```python
from build123d import *

# Parameters (mm, degrees)
SKETCH1_W                = 71
SKETCH1_H                = 80
BOSS_EXTRUDE1_DEPTH      = 10
SKETCH3_W                = 10
SKETCH3_H                = 10
CUT_EXTRUDE1_DEPTH       = 10
SKETCH5_W                = 28.158683969
SKETCH5_H                = 10
CUT_EXTRUDE3_DEPTH       = 10
CIRPATTERN1_COUNT        = 3
M6_CLEARANCE_HOLE1_D     = 6.3
CUT_EXTRUDE6_DEPTH       = 3
SKETCH11_R               = 1.55
CUT_EXTRUDE7_DEPTH       = 108.429046352
CIRPATTERN2_COUNT        = 3
CUT_EXTRUDE8_DEPTH       = 10
CUT_EXTRUDE9_DEPTH       = 10
CUT_EXTRUDE10_DEPTH      = 10
SKETCH15_W               = 111
SKETCH15_H               = 42
BOSS_EXTRUDE2_DEPTH      = 10
SKETCH22_W               = 15
SKETCH22_H               = 54
BOSS_EXTRUDE3_DEPTH      = 10
M4_CLEARANCE_HOLE1_D     = 4.5
M4_CLEARANCE_HOLE1_DEPTH = 30
M4_CLEARANCE_HOLE1_TIP   = 1.351936393
SKETCH26_W               = 47.7
SKETCH26_H               = 6
CUT_EXTRUDE13_DEPTH      = 10
CHAMFER1_SIZE            = 4
CHAMFER1_SIZE_2          = 6.92820323
SKETCH27_W               = 6.3
SKETCH27_H               = 6
CUT_EXTRUDE14_DEPTH      = 10
CHAMFER2_SIZE            = 6.92820323
CHAMFER2_SIZE_2          = 4
CUT_EXTRUDE15_DEPTH      = 10
CUT_EXTRUDE16_DEPTH      = 2.2
CUT_EXTRUDE17_DEPTH      = 10
M4_CLEARANCE_HOLE2_D     = 4.5
SKETCH33_W               = 30
SKETCH33_H               = 90
CUT_EXTRUDE18_DEPTH      = 138.189649755
SKETCH34_W               = 10
SKETCH34_H               = 22
BOSS_EXTRUDE4_DEPTH      = 5
SKETCH38_R               = 2.25
CUT_EXTRUDE20_DEPTH      = 41
CHAMFER3_SIZE            = 2


with BuildPart() as part:
    # Sketch1 → Boss-Extrude1 (new body)
    with BuildSketch(Plane.XY):
        with Locations((35.5, 40)):
            Rectangle(SKETCH1_W, SKETCH1_H)
    extrude(amount=BOSS_EXTRUDE1_DEPTH)

    # Sketch3 → Cut-Extrude1 (cut)
    with BuildSketch(Plane.XY.offset(10)):
        Polygon((25.580127019, 57.655444566), (16.919872981, 52.655444566), (11.919872981, 61.315698604), (20.580127019, 66.315698604), align=None)
        Polygon((11.919872981, 18.684301396), (20.580127019, 13.684301396), (25.580127019, 22.344555434), (16.919872981, 27.344555434), align=None)
        with Locations((52.5, 40)):
            Rectangle(SKETCH3_W, SKETCH3_H)
    extrude(amount=-CUT_EXTRUDE1_DEPTH, mode=Mode.SUBTRACT)

    # Sketch5 → Cut-Extrude3 (cut)
    with BuildSketch(Plane.XY.offset(10)):
        with Locations((71.579341985, 40)):
            Rectangle(SKETCH5_W, SKETCH5_H)
    cut_extrude3 = extrude(amount=-CUT_EXTRUDE3_DEPTH, mode=Mode.SUBTRACT)

    # CirPattern1: Cut-Extrude3 ×3 about axis
    cirpattern1_axis = Axis((30, 40, 10), (0, 0, -1))
    for i in range(1, CIRPATTERN1_COUNT):
        add(cut_extrude3.rotate(cirpattern1_axis, i * 360 / CIRPATTERN1_COUNT), mode=Mode.SUBTRACT)

    # M6 Clearance Hole1 (through all)
    with Locations(Plane.XY.offset(10)):
        with Locations((30, 40)):
            Hole(M6_CLEARANCE_HOLE1_D / 2)

    # Sketch10 → Cut-Extrude6 (cut)
    with BuildSketch(Plane.XY.offset(10)):
        Polygon((30, 45.773502692), (25, 42.886751346), (25, 37.113248654), (30, 34.226497308), (35, 37.113248654), (35, 42.886751346), align=None)
    extrude(amount=-CUT_EXTRUDE6_DEPTH, mode=Mode.SUBTRACT)

    # Sketch11 → Cut-Extrude7 (cut, through all)
    with BuildSketch(Plane.XZ):
        with Locations(Location((62.5, 5, 0), (0, 0, 270))):
            Circle(SKETCH11_R)
    cut_extrude7 = extrude(amount=-CUT_EXTRUDE7_DEPTH, mode=Mode.SUBTRACT)

    # CirPattern2: Cut-Extrude7 ×3 about axis
    cirpattern2_axis = Axis((30, 40, 7), (0, 0, 1))
    for i in range(1, CIRPATTERN2_COUNT):
        add(cut_extrude7.rotate(cirpattern2_axis, i * 360 / CIRPATTERN2_COUNT), mode=Mode.SUBTRACT)

    # Sketch12 → Cut-Extrude8 (cut)
    with BuildSketch(Plane.XY.offset(10)):
        Polygon((71, 0), (71, 25), (38.660254038, 25), (24.226497308, 0), align=None)
    cut_extrude8 = extrude(amount=-CUT_EXTRUDE8_DEPTH, mode=Mode.SUBTRACT)

    # Mirror1: Cut-Extrude8 across plane
    add(cut_extrude8.mirror(Plane(origin=(0, 40, 0), x_dir=(0, 0, 1), z_dir=(0, -1, 0))), mode=Mode.SUBTRACT)

    # Sketch13 → Cut-Extrude9 (cut)
    with BuildSketch(Plane.XY.offset(10)):
        Polygon((0, 61.961524227), (8.624364028, 47.023687548), (8.624364028, 32.976312452), (0, 18.038475773), align=None)
    extrude(amount=-CUT_EXTRUDE9_DEPTH, mode=Mode.SUBTRACT)

    # Sketch14 → Cut-Extrude10 (cut)
    with BuildSketch(Plane.XY.offset(10)):
        Polygon((-3.240381057, 12.425971147), (22.740381057, -2.574028853), (18.169872981, -10.490381057), (-7.810889132, 4.509618943), align=None)
    cut_extrude10 = extrude(amount=-CUT_EXTRUDE10_DEPTH, mode=Mode.SUBTRACT)

    # Mirror2: Cut-Extrude10 across plane
    add(cut_extrude10.mirror(Plane(origin=(0, 40, 0), x_dir=(0, 0, 1), z_dir=(0, -1, 0))), mode=Mode.SUBTRACT)

    # Sketch15 → Boss-Extrude2 (add)
    with BuildSketch(Plane.XY.offset(10)):
        with Locations((126.5, 40)):
            Rectangle(SKETCH15_W, SKETCH15_H)
    extrude(amount=-BOSS_EXTRUDE2_DEPTH)

    # Sketch22 → Boss-Extrude3 (add)
    with BuildSketch(Plane.XY.offset(10)):
        with Locations((174.5, 40)):
            Rectangle(SKETCH22_W, SKETCH22_H)
    extrude(amount=-BOSS_EXTRUDE3_DEPTH)

    # M4 Clearance Hole1
    with Locations(Plane(origin=(182, 0, 0), x_dir=(0, 0, -1), z_dir=(1, 0, 0))):
        with Locations((-5, 62.5), (-5, 17.5)):
            Hole(M4_CLEARANCE_HOLE1_D / 2, depth=M4_CLEARANCE_HOLE1_DEPTH)
            with Locations((0, 0, -(M4_CLEARANCE_HOLE1_DEPTH + M4_CLEARANCE_HOLE1_TIP / 2))):  # 118° drill point
                Cone(0, M4_CLEARANCE_HOLE1_D / 2, M4_CLEARANCE_HOLE1_TIP, mode=Mode.SUBTRACT)

    # Sketch26 → Cut-Extrude13 (cut)
    with BuildSketch(Plane.XY.offset(10)):
        with Locations((143.15, 58)):
            Rectangle(SKETCH26_W, SKETCH26_H)
    cut_extrude13 = extrude(amount=-CUT_EXTRUDE13_DEPTH, mode=Mode.SUBTRACT)

    # Mirror3: Cut-Extrude13 across plane
    add(cut_extrude13.mirror(Plane(origin=(0, 40, 0), x_dir=(0, 0, 1), z_dir=(0, -1, 0))), mode=Mode.SUBTRACT)

    # Chamfer1
    # the kernel refuses this chamfer: 6.92820323, 4 mm, written as the material it adds along each edge
    with BuildSketch(Plane(origin=(119.3, 25, 10), x_dir=(0.9983227437537926, 0.05789386240267157, 0), z_dir=(0, 0, -1))) as chamfer1_piece_1_section:
        Polygon((CHAMFER1_SIZE * 0.998322743754, CHAMFER1_SIZE * 0.0578938624027), (-CHAMFER1_SIZE_2 * 0.057893862405, CHAMFER1_SIZE_2 * 0.998322743793), (0, 0), align=None)
    chamfer1_piece_1 = extrude(amount=10, mode=Mode.PRIVATE)
    chamfer1_piece_1 = split(chamfer1_piece_1, bisect_by=Plane(origin=(120.625811149, 19, 5), z_dir=(0, 1, 0)), keep=Keep.TOP, mode=Mode.PRIVATE)
    add(chamfer1_piece_1)
    with BuildSketch(Plane(origin=(119.3, 55, 10), x_dir=(-0.019326765612697788, 0.999813220622208, 0), z_dir=(0, 0, -1))) as chamfer1_piece_2_section:
        Polygon((CHAMFER1_SIZE_2 * 0.999813220662, CHAMFER1_SIZE_2 * 0.0193267656135), (-CHAMFER1_SIZE * 0.0193267656127, CHAMFER1_SIZE * 0.999813220622), (0, 0), align=None)
    chamfer1_piece_2 = extrude(amount=10, mode=Mode.PRIVATE)
    chamfer1_piece_2 = split(chamfer1_piece_2, bisect_by=Plane(origin=(120.625811149, 61, 5), z_dir=(0, -1, 0)), keep=Keep.TOP, mode=Mode.PRIVATE)
    add(chamfer1_piece_2)

    # Sketch27 → Cut-Extrude14 (cut)
    with BuildSketch(Plane.XY.offset(10)):
        with Locations((74.15, 58)):
            Rectangle(SKETCH27_W, SKETCH27_H)
    cut_extrude14 = extrude(amount=-CUT_EXTRUDE14_DEPTH, mode=Mode.SUBTRACT)

    # Mirror4: Cut-Extrude14 across plane
    add(cut_extrude14.mirror(Plane(origin=(0, 40, 0), x_dir=(0, 0, 1), z_dir=(0, -1, 0))), mode=Mode.SUBTRACT)

    # Chamfer2
    # the kernel refuses this chamfer: 6.92820323, 4 mm, written as the material it adds along each edge
    with BuildSketch(Plane(origin=(77.3, 55, 10), x_dir=(0.019326765612699692, 0.9998132206222079, 0), z_dir=(0, 0, -1))) as chamfer2_piece_1_section:
        Polygon((CHAMFER2_SIZE * 0.999813220662, -CHAMFER2_SIZE * 0.0193267656135), (-CHAMFER2_SIZE_2 * 0.0193267656127, -CHAMFER2_SIZE_2 * 0.999813220622), (0, 0), align=None)
    chamfer2_piece_1 = extrude(amount=10, mode=Mode.PRIVATE)
    chamfer2_piece_1 = split(chamfer2_piece_1, bisect_by=Plane(origin=(75.974188851, 61, 5), z_dir=(0, -1, 0)), keep=Keep.TOP, mode=Mode.PRIVATE)
    add(chamfer2_piece_1)
    with BuildSketch(Plane(origin=(77.3, 25, 10), x_dir=(-0.9983227437537929, 0.05789386240266474, 0), z_dir=(0, 0, -1))) as chamfer2_piece_2_section:
        Polygon((CHAMFER2_SIZE_2 * 0.998322743754, -CHAMFER2_SIZE_2 * 0.0578938624027), (-CHAMFER2_SIZE * 0.057893862405, -CHAMFER2_SIZE * 0.998322743793), (0, 0), align=None)
    chamfer2_piece_2 = extrude(amount=10, mode=Mode.PRIVATE)
    chamfer2_piece_2 = split(chamfer2_piece_2, bisect_by=Plane(origin=(75.974188851, 19, 5), z_dir=(0, 1, 0)), keep=Keep.TOP, mode=Mode.PRIVATE)
    add(chamfer2_piece_2)

    # Sketch21 → Cut-Extrude15 (cut)
    with BuildSketch(Plane.XY.offset(10)):
        with BuildLine():
            Line((97.55, 47.5), (99.05, 47.5))
            ThreePointArc((99.05, 47.5), (106.55, 40), (99.05, 32.5))
            Line((99.05, 32.5), (97.55, 32.5))
            ThreePointArc((97.55, 32.5), (90.05, 40), (97.55, 47.5))
        make_face()
    extrude(amount=-CUT_EXTRUDE15_DEPTH, mode=Mode.SUBTRACT)

    # Sketch28 → Cut-Extrude16 (cut)
    with BuildSketch(Plane.XY.offset(10)):
        with BuildLine():
            Line((97.55, 51.25), (99.05, 51.25))
            ThreePointArc((99.05, 51.25), (110.3, 40), (99.05, 28.75))
            Line((99.05, 28.75), (97.55, 28.75))
            ThreePointArc((97.55, 28.75), (86.3, 40), (97.55, 51.25))
        make_face()
    extrude(amount=-CUT_EXTRUDE16_DEPTH, mode=Mode.SUBTRACT)

    # Sketch29 → Cut-Extrude17 (cut)
    with BuildSketch(Plane.XY.offset(10)):
        with BuildLine():
            Line((82.05, 57.2), (83.55, 57.2))
            ThreePointArc((83.55, 57.2), (85.25, 55.5), (83.55, 53.8))
            Line((83.55, 53.8), (82.05, 53.8))
            ThreePointArc((82.05, 53.8), (80.35, 55.5), (82.05, 57.2))
        make_face()
        with BuildLine():
            Line((113.05, 53.8), (114.55, 53.8))
            ThreePointArc((114.55, 53.8), (116.25, 55.5), (114.55, 57.2))
            Line((114.55, 57.2), (113.05, 57.2))
            ThreePointArc((113.05, 57.2), (111.35, 55.5), (113.05, 53.8))
        make_face()
        with BuildLine():
            Line((113.05, 22.8), (114.55, 22.8))
            ThreePointArc((114.55, 22.8), (116.25, 24.5), (114.55, 26.2))
            Line((114.55, 26.2), (113.05, 26.2))
            ThreePointArc((113.05, 26.2), (111.35, 24.5), (113.05, 22.8))
        make_face()
        with BuildLine():
            Line((82.05, 22.8), (83.55, 22.8))
            ThreePointArc((83.55, 22.8), (85.25, 24.5), (83.55, 26.2))
            Line((83.55, 26.2), (82.05, 26.2))
            ThreePointArc((82.05, 26.2), (80.35, 24.5), (82.05, 22.8))
        make_face()
    extrude(amount=-CUT_EXTRUDE17_DEPTH, mode=Mode.SUBTRACT)

    # M4 Clearance Hole2 (through all)
    with Locations(Plane.XY.offset(10)):
        with Locations((134, 50.5), (155, 50.5), (155, 29.5), (134, 29.5)):
            Hole(M4_CLEARANCE_HOLE2_D / 2)

    # Sketch33 → Cut-Extrude18 (cut, through all)
    with BuildSketch(Plane.ZY.offset(-71)):
        with Locations((5, 40)):
            Rectangle(SKETCH33_W, SKETCH33_H)
    extrude(amount=-CUT_EXTRUDE18_DEPTH, mode=Mode.SUBTRACT)

    # Sketch34 → Boss-Extrude4 (add)
    with BuildSketch(Plane(origin=(71, 0, 0), x_dir=(0, 0, -1), z_dir=(1, 0, 0))):
        with Locations((-5, 56)):
            Rectangle(SKETCH34_W, SKETCH34_H)
    boss_extrude4 = extrude(amount=-BOSS_EXTRUDE4_DEPTH)

    # Mirror5: Boss-Extrude4 across plane
    add(boss_extrude4.mirror(Plane(origin=(0, 40, 0), x_dir=(0, 0, 1), z_dir=(0, -1, 0))))

    # Sketch38 → Cut-Extrude20 (cut)
    with BuildSketch(Plane(origin=(71, 0, 0), x_dir=(0, 0, -1), z_dir=(1, 0, 0))):
        with Locations((-5, 62.5)):
            Circle(SKETCH38_R)
        with Locations((-5, 17.5)):
            Circle(SKETCH38_R)
    extrude(amount=-CUT_EXTRUDE20_DEPTH, mode=Mode.SUBTRACT)

    # Chamfer3
    chamfer3_edges = [part.edges().sort_by_distance(p)[0] for p in [
        (68.5, 67, 10),
        (68.5, 67, 0),
        (68.5, 13, 10),
        (68.5, 13, 0),
    ]]
    chamfer(chamfer3_edges, length=CHAMFER3_SIZE)


solid = part.part
```
The model under review builds one solid part; all positions refer to its coordinate system, in mm. A direction names the side the tool comes from. Round coordinates to 2 decimals unless told otherwise and drop trailing zeros. Order: outer loops, then holes, each group sorted by start corner. A loop starts at its lowest first (then second) coordinate and runs counter-clockwise, first axis right, second up. Notation, with made-up numbers: (-15, -37.75) -> (11, -37.75) arc R29 ccw to (11, -6.75) -> close; hole circle Ø7 at (57.25, 16). An arc over 180 degrees is marked (long way). One line per item, written item: value. Start each with the question number.
Q1. Wall thickness on line 1 (Y direction, x = 67.5, z = 5); line 2 (X direction, y = 20.5, z = 5.25); line 3 (Y direction, x = 16.5, z = 1): over which ranges is each line inside the solid? List them lowest first.
Q2. Machinability: for faces 4 (the face through (31.54, 12.67, 5.07)), 5 (the face through (32.535, 44.31, 8.521)), 6 (the face through (32.24, 19.73, 5.29)), 7 (the face through (4.25, 54.6, 5.07)), which of the approach directions +Z, -Z, +X, -X, +Y, -Y give a long, thin tool a straight path to every point of the face, cutting with its end or side? Answer none if there is none.
Q3. Take a section at B-B (y = 41). Write out the cut boundary in (x, z), and give its area (3 significant figures).
Q4. Take a section at C-C (x = 29). Write out the cut boundary in (y, z).
Q5. Take a section at A-A (x = 56). Write out the cut boundary in (y, z), and give its area (3 significant figures).
Q6. Mouldability with a two-part tool opening along X and no side actions: class faces 1 (the face through (0, 14, 5)), 2 (the face through (69, 67, 5)), 3 (the face through (31.544, 67.325, 5.07)) as released by +X, released by -X, zero draft, split by the parting line, or undercut.
Q7. Clearance check with flat-ended pins moving along their axes: pin 1 Ø7 at (x, y) = (30, 40) entering from +Z; pin 2 Ø1.3 at (y, z) = (17.5, 5) entering from +X; pin 3 Ø2 at (x, z) = (28.5, 1) entering from +Y. State where each tip first meets the part, or that it passes through.
Reported:
1. line 1: y = 13 to 15.25, 19.75 to 35, 45 to 60.25, 64.75 to 67
1. line 2: x = 1.83 to 12.97, 24.52 to 36.06, 66 to 71
1. line 3: y = 1.03 to 6.62, 26.62 to 53.38, 73.38 to 78.97
2. face 4: +Z, -Z, -Y
2. face 5: +Z
2. face 6: +X
2. face 7: +Z, -Z, -X
3. outline: (8.62, 0) -> (27.01, 0) -> (27.01, 7) -> (25, 7) -> (25, 10) -> (8.62, 10) -> close; (32.99, 0) -> (47.5, 0) -> (47.5, 10) -> (35, 10) -> (35, 7) -> (32.99, 7) -> close
3. area: 317 mm2
4. outline: (8.27, 0) -> (37.01, 0) -> (37.01, 7) -> (34.8, 7) -> (34.8, 10) -> (8.27, 10) -> close; (42.99, 0) -> (71.73, 0) -> (71.73, 10) -> (45.2, 10) -> (45.2, 7) -> (42.99, 7) -> close
5. outline: (25, 0) -> (35, 0) -> (35, 10) -> (25, 10) -> close; (45, 0) -> (55, 0) -> (55, 10) -> (45, 10) -> close
5. area: 200 mm2
6. face 1: released by -X
6. face 2: zero draft
6. face 3: undercut
7. pin 1: stops at z = 7
7. pin 2: stops at x = 30
7. pin 3: stops at y = 74.33
